The model under review builds one solid part; all positions refer to its coordinate system, in mm. A direction names the side the tool comes from. Coordinates: 2 decimals unless noted, no trailing zeros. Loops run counter-clockwise (first coordinate to the right, second up) from the corner with the lowest first, then second, coordinate; pieces in that order, holes last. Notation, with made-up numbers: (-15, -34) - (26, -34) arc R32 ccw to (26, -3) - close; hole circle Ø3 at (29, -20). An arc over 180 degrees is marked (long way). Use a Markdown table: item, result. Add a question column.
1) For faces 4 (the flat face through (14, 10, 7)), 5 (the cylindrical face through (23.146, 0.676, 3.549)), list the 3-axis set-ups (+Z, -Z, +X, -X, +Y, -Y) from which the entire face can be reached by the end or side of a thin tool; tool diameter is ignored.
2) Add section A-A, the plane z = 1.75. Give the boundary of the cut face in (x, y).
3) The part is to be moulded in two halves that separate along Y. For faces 1 (the flat face through (-14.7, -15, 3.5)), 2 (the cylindrical face through (-0.488, -23.196, 3.549)), 3 (the flat face through (-26.87, 0, 4)), say which applies: pulls with the +Y half, pulls with the -Y half, needs draft (parallel to the pull), parting line crosses it, or undercut.
4) Add section B-B, the plane x = 0. Give the boundary of the cut face in (y, z), and give its area (3 significant figures).
5) To check wall thickness, follow L1, parallel to Y at x = 0, z = 1.75; L2, parallel to Y at x = -1, z = 4.75; L3, parallel to Z at x = -2, y = 18.5. State the ranges of each line that lie inside material, in increasing order. Write a range as [from, to].
6) Add section D-D, the plane y = -21. Give the boundary of the cut face in (x, z), and give its area (3 significant figures).
7) Clearance check with flat-ended pins moving along their axes: pin 1 (1.5 mm diameter, centred on x = 0.5, y = -10.5, fed in from -Z); pin 2 (6 mm diameter, centred on x = 0, y = -21, fed in from +Z); pin 3 (4 mm diameter, centred on x = 6, z = 4.5, fed in from +Y); pin 4 (3 mm diameter, centred on y = 18, z = 6, fed in from -X). State where each tip first meets the part, or that it passes through.
Autodesk Inventor part; units mm, degrees
ref_plane "YZ Plane" through (0, 0, 0) normal (1, 0, 0) x (0, 1, 0)
ref_plane "XZ Plane" through (0, 0, 0) normal (0, 1, 0) x (-1, 0, 0)
ref_plane "XY Plane" through (0, 0, 0) normal (0, 0, 1) x (1, 0, 0)
sketch "Sketch1" plane through (0, 0, 0) normal (0, 0, 1) x (1, 0, 0)
  circle A0 centre (0, 0) radius 17 construction
  circle A1 centre (0, 0) radius 6 construction
  line L0 (-29.6985, 0) -> (0, 29.6985)
  line L1 (0, 29.6985) -> (29.6985, 0)
  line L2 (29.6985, 0) -> (0, -29.6985)
  line L3 (0, -29.6985) -> (-29.6985, 0)
  line L4 (-29.6985, 0) -> (29.6985, 0) construction
  line L5 (0, 29.6985) -> (0, -29.6985) construction
  point P0 (0, 21)
  point P1 (21, 0)
  point P2 (-21, 0)
  point P3 (0, -21)
  dimension "d0" = 34
  dimension "d1" = 12
  dimension "d2" = 21
  dimension "d3" = 21
  dimension "d4" = 21
  dimension "d5" = 21
  dimension "d6" = 21
  dimension "d7" = 42
  dimension "d8" = 42
extrude "Extrusion1" add sketch "Sketch1" along normal blind 7
sketch "Sketch2" plane through (0, 0, 7) normal (0, 0, 1) x (1, 0, 0)
  circle A0 centre (0, 0) radius 6
  circle A1 centre (0, 0) radius 18
  circle A2 centre (0, 21) radius 2.25
  circle A3 centre (21, 0) radius 2.25
  circle A4 centre (0, -21) radius 2.25
  circle A5 centre (-21, 0) radius 2.25
  dimension "d11" = 12
  dimension "d12" = 36
  dimension "d13" = 4.5
  dimension "d14" = 4.5
  dimension "d15" = 4.5
  dimension "d16" = 4.5
  dimension "d17" = 21
  dimension "d18" = 21
  dimension "d19" = 21
  dimension "d20" = 21
extrude "Extrusion2" cut sketch "Sketch2" against normal blind 20 contours A2 | A3 | A4 | A5
sketch "Sketch3" plane through (0, 0, 7) normal (0, 0, 1) x (1, 0, 0)
  circle A0 centre (0, 0) radius 17
  circle A1 centre (0, 0) radius 6
  dimension "d23" = 34
  dimension "d24" = 12
extrude "Extrusion3" cut sketch "Sketch3" against normal blind 20 contours A1
sketch "Sketch4" plane through (0, 0, 7) normal (0, 0, 1) x (1, 0, 0)
  circle A0 centre (0, 0) radius 6
  circle A1 centre (0, 0) radius 17
  dimension "d27" = 34
extrude "Extrusion4" add sketch "Sketch4" along normal blind 8
chamfer "Chamfer1" distance 4 angle 45 1 edges at (0, 29.6985, 3.5)
chamfer "Chamfer2" distance 4 angle 45 1 edges at (29.6985, 0, 3.5)
chamfer "Chamfer3" distance 4 angle 45 1 edges at (-29.6985, 0, 3.5)
chamfer "Chamfer4" distance 4 angle 45 1 edges at (0, -29.6985, 3.5)
equation "\"d14\" = d13"
equation "\"d15\" = d13"
equation "\"d16\" = d13"
equation "\"d18\" = d17"
equation "\"d19\" = d17"
properties part number "ff12"
From the geometry:
| question | item | result |
|---|---|---|
| 1 | face 4 | +Z |
| 1 | face 5 | +Z, -Z |
| 2 | outline | (-26.87, -2.83) - (-2.83, -26.87) - (2.83, -26.87) - (26.87, -2.83) - (26.87, 2.83) - (2.83, 26.87) - (-2.83, 26.87) - (-26.87, 2.83) - close; hole circle Ø4.5 at (-21, 0); hole circle Ø12 at (0, 0); hole circle Ø4.5 at (0, -21); hole circle Ø4.5 at (0, 21); hole circle Ø4.5 at (21, 0) |
| 3 | face 1 | pulls with the -Y half |
| 3 | face 2 | undercut |
| 3 | face 3 | needs draft |
| 4 | outline | (-26.87, 0) - (-23.25, 0) - (-23.25, 7) - (-26.87, 7) - close; (-18.75, 0) - (-6, 0) - (-6, 15) - (-17, 15) - (-17, 7) - (-18.75, 7) - close; (6, 0) - (18.75, 0) - (18.75, 7) - (17, 7) - (17, 15) - (6, 15) - close; (23.25, 0) - (26.87, 0) - (26.87, 7) - (23.25, 7) - close |
| 4 | area | 405 mm^2 |
| 5 | L1 | y = [-26.87, -23.25], [-18.75, -6], [6, 18.75], [23.25, 26.87] |
| 5 | L2 | y = [-26.87, -23.02], [-18.98, -5.92], [5.92, 18.98], [23.02, 26.87] |
| 5 | L3 | z = [0, 7] |
| 6 | outline | (-8.7, 0) - (-2.25, 0) - (-2.25, 7) - (-8.7, 7) - close; (2.25, 0) - (8.7, 0) - (8.7, 7) - (2.25, 7) - close |
| 6 | area | 90.3 mm^2 |
| 7 | pin 1 | stops at z = 0 |
| 7 | pin 2 | stops at z = 7 |
| 7 | pin 3 | stops at y = 25.7 |
| 7 | pin 4 | stops at x = -13.2 |
